from build123d import *

# Parameters (mm, degrees)
F0_R          = 63.5
F1_DEPTH      = 279.4
F2_T          = -12.7
F3_R          = 6.35
F4_DEPTH      = 279.401
F6_DEPTH      = 50.8
F7_R          = 6.35
F7_R_2        = 3.81
F8_DEPTH      = 25.4
F8_DEPTH_BACK = 5.08
F9_R          = 12.7


with BuildPart() as f1:
    # F0 (on Top) → F1 (new body)
    with BuildSketch(Plane.XY):
        with Locations((-64.736634, 44.41886)):
            Circle(F0_R)
    extrude(amount=F1_DEPTH)

    # F2
    f2_openings = [f1.faces().sort_by_distance(p)[0] for p in [
        (-64.736634, 44.41886, 279.4),
    ]]
    offset(amount=F2_T, openings=f2_openings)

    # F3 (on face) → F4 (cut, through all)
    with BuildSketch(Plane(origin=(0, 0, 0), x_dir=(1, 0, 0), z_dir=(0, 0, -1))):
        with Locations((-26.847913, -40.412018)):
            Circle(F3_R)
    extrude(amount=-F4_DEPTH, mode=Mode.SUBTRACT)

    # F5 (on Right) → F6 (cut)
    with BuildSketch(Plane.YZ):
        with BuildLine():
            ThreePointArc((44.45, 62.627283), (39.959872, 51.787155), (50.8, 56.277283))
            ThreePointArc((50.8, 56.277283), (48.940128, 60.767411), (44.45, 62.627283))
        make_face()
        with BuildLine():
            ThreePointArc((50.8, 246.777283), (39.959872, 251.267411), (44.45, 240.427283))
            ThreePointArc((44.45, 240.427283), (48.940128, 242.287155), (50.8, 246.777283))
        make_face()
    extrude(amount=-F6_DEPTH, mode=Mode.SUBTRACT)

    # F7 (on Right) → F8 (join, two sides)
    with BuildSketch(Plane.YZ) as f8_sk:
        with Locations((44.45, 246.777283)):
            Circle(F7_R)
        with Locations((44.45, 246.777283)):
            Circle(F7_R_2, mode=Mode.SUBTRACT)
        with Locations((44.45, 56.277283)):
            Circle(F7_R)
        with Locations((44.45, 56.277283)):
            Circle(F7_R_2, mode=Mode.SUBTRACT)
    extrude(amount=F8_DEPTH)
    extrude(f8_sk.sketch, amount=-F8_DEPTH_BACK)

    # F9
    f9_edges = [f1.edges().sort_by_distance(p)[0] for p in [
        (-128.236634, 44.41886, 0),
    ]]
    fillet(f9_edges, radius=F9_R)


solid = f1.part
Geometry: final body of the model. Coordinates: model frame, mm. A direction names the side the tool comes from. Give positions to 0.01 mm unless a question says otherwise; leave off trailing zeros. Write each loop counter-clockwise with the first axis right and the second up, starting at its lowest first coordinate (ties: lowest second). Pieces come first, ordered by that corner, then holes.
(1) First-contact query: P1, Ø4, axis at y = 52.5, z = 75, coming from the +X side; P2, Ø14.5, axis at x = -26.85, y = 40.41, coming from the +Z side; P3, Ø7.5, axis at y = 44.45, z = 56.28, coming from the +X side. Flat tips, straight axial feed; report the tip coordinate or a pass-through.
(2) Mould query, pull axis X, two halves, no side actions, for faces 1 (the cylindrical face through (-111.539, 87.335, 144.183)), 2 (the cylindrical face through (12.11, 47.38, 241.144)), 3 (the cylindrical face through (-16.282, 59.678, 144.183)). Classes: released by +X, released by -X, zero draft, split by the parting line, or undercut.
(3) Ray query, line 1 (Z direction, x = -8, y = 44); line 2 (X direction, y = 44, z = 27); line 3 (Z direction, x = -10, y = 44). Return the intervals inside material, ascending.
(4) Cut plane B-B, the plane z = 134. Return loops of the section in (x, y).
(5) Cut plane A-A, the plane x = 4. Return loops of the section in (y, z).
(6) Access query for faces 4 (the cylindrical face through (-20.791, 38.505, 6.261)), 5 (the cylindrical face through (9.95, 41.64, 58.85)), 6 (the flat face through (25.4, 49, 247)), 7 (the flat face through (-65, 45, 12.7)), 8 (the flat face through (-5.08, 44, 52)). Directions: +Z, -Z, +X, -X, +Y, -Y. A direction counts if a zero-diameter tool reaches every point of the face in a straight line with its end or side. Return the directions, or none.
Values follow:
1. P1: stops at x = -1.53
1. P2: stops at z = 12.7
1. P3: stops at x = -115.4
2. face 1: split by the parting line
2. face 2: zero draft
2. face 3: undercut
3. line 1: z = 1.47 to 49.94, 62.61 to 240.44, 253.11 to 279.4
3. line 2: x = -128.24 to -115.53, -13.94 to -1.24
3. line 3: z = 0.63 to 49.94, 62.61 to 240.44, 253.11 to 279.4
4. outline: circle Ø127 at (-64.74, 44.42); hole circle Ø101.6 at (-64.74, 44.42)
5. outline: circle Ø12.7 at (44.45, 56.28); circle Ø12.7 at (44.45, 246.78); hole circle Ø7.62 at (44.45, 56.28); hole circle Ø7.62 at (44.45, 246.78)
6. face 4: +Z, -Z
6. face 5: +X
6. face 6: +Z, -Z, +X, +Y, -Y
6. face 7: +Z
6. face 8: none
